```python
from build123d import *

# Parameters (mm, degrees)
F1_DEPTH = 25.4
F2_R     = 6.35
F3_DEPTH = 52.07
F5_DEPTH = 48.768
F7_DEPTH = 25.4
F9_DEPTH = 25.4


with BuildPart() as f1:
    # F0 (on Front) → F1 (new body)
    with BuildSketch(Plane.XZ):
        Polygon((0, 38.1), (0, 0), (76.2, 0), (76.2, 12.7), (25.4, 12.7), (25.4, 38.1), align=None)
    extrude(amount=-F1_DEPTH)

    # F2 (on face) → F3 (cut)
    with BuildSketch(Plane.XZ):
        with Locations((12.7231444902, 26.1663774417)):
            Circle(F2_R)
    extrude(amount=-F3_DEPTH, mode=Mode.SUBTRACT)

    # F4 (on face) → F5 (cut)
    with BuildSketch(Plane.XZ):
        with BuildLine():
            ThreePointArc((12.7, 38.1), (21.6802561211, 34.3802561211), (25.4, 25.4))
            Line((25.4, 25.4), (25.4, 38.1))
            Line((25.4, 38.1), (12.7, 38.1))
        make_face()
        with BuildLine():
            ThreePointArc((0, 25.4), (3.7197438789, 34.3802561211), (12.7, 38.1))
            Line((12.7, 38.1), (0, 38.1))
            Line((0, 38.1), (0, 25.4))
        make_face()
    extrude(amount=-F5_DEPTH, mode=Mode.SUBTRACT)

    # F6 (on face) → F7 (cut)
    with BuildSketch(Plane.XY.offset(12.7)):
        with BuildLine():
            Line((63.5, 19.05), (38.1, 19.05))
            ThreePointArc((38.1, 19.05), (31.75, 12.7), (38.1, 6.35))
            Line((38.1, 6.35), (63.5, 6.35))
            ThreePointArc((63.5, 6.35), (69.85, 12.7), (63.5, 19.05))
        make_face()
    extrude(amount=-F7_DEPTH, mode=Mode.SUBTRACT)

    # F8 (on face) → F9 (cut)
    with BuildSketch(Plane.XY.offset(12.7)):
        with BuildLine():
            ThreePointArc((63.5, 25.4), (72.4802561211, 21.6802561211), (76.2, 12.7))
            Line((76.2, 12.7), (76.2, 25.4))
            Line((76.2, 25.4), (63.5, 25.4))
        make_face()
        with BuildLine():
            ThreePointArc((76.2, 12.7), (72.4802561211, 3.7197438789), (63.5, 0))
            Line((63.5, 0), (76.2, 0))
            Line((76.2, 0), (76.2, 12.7))
        make_face()
    extrude(amount=-F9_DEPTH, mode=Mode.SUBTRACT)


solid = f1.part
```
Here's how the part is built. I have some questions about the finished solid (model axes, mm). A direction names the side the tool comes from. Round coordinates to 2 decimals unless told otherwise and drop trailing zeros. Write each loop counter-clockwise with the first axis right and the second up, starting at its lowest first coordinate (ties: lowest second). Pieces come first, ordered by that corner, then holes. Notation, with made-up numbers: M -5.5,-17 L 46.5,-17 A22 ccw 46.5,-5 Z; hole C -38.5,-16 d8. An arc over 180 degrees is marked long. Answer as CSV lines item,"result". Start each with the question number.
1. Suppose I cut it at A-A on y = 16.75. Write out the boundary of the cut face in (x, z), then the cut area to 3 significant figures.
2. Suppose I cut it at D-D on y = 4.25. Write out the boundary of the cut face in (x, z).
3. I need wall thicknesses on probe 1 along Y at (x, z) = (49, 8.5); probe 2 along Z at (x, y) = (12, 4); probe 3 along X at (y, z) = (20.75, 28). Which ranges of each line are inside material? Lowest first, please.
4. Thinking about a two-plate mould opening in X: for faces 1 (the cylindrical face through (69.85, 12.56, 6.44)), 2 (the flat face through (25.4, 13, 19)), 3 (the flat face through (29, 13, 0)), which applies, released by +X, released by -X, zero draft, split by the parting line, or undercut?
5. On a 3-axis mill with a long thin cutter (end or side, diameter ignored), from which of +Z, -Z, +X, -X, +Y, -Y can I reach the whole of each face in a straight line? I mean faces 4 (the flat face through (51, 4, 12.7)), 5 (the flat face through (51, 19.05, 6)), 6 (the flat face through (24, 0, 15)). Say none if no direction works.
6. Suppose I cut it at C-C on z = 10. Write out the boundary of the cut face in (x, y).
7. Suppose I cut it at B-B on x = 49. Write out the boundary of the cut face in (y, z).
8. I'm going to push flat-ended pins straight in: pin 1 Ø14.5 at (x, z) = (12.72, 26.17) entering from +Y; pin 2 Ø12.5 at (x, y) = (42, 15.5) entering from +Z. Where does each tip first touch, or does it pass through?
Check result:
1,outline,"M 0,0 L 33.21,0 L 33.21,12.7 L 25.4,12.7 L 25.4,25.4 A12.7 ccw 0,25.4 Z; M 68.39,0 L 75.54,0 L 75.54,12.7 L 68.39,12.7 Z; hole C 12.72,26.17 d12.7"
1,area,"962 mm2"
2,outline,"M 0,0 L 72.98,0 L 72.98,12.7 L 25.4,12.7 L 25.4,25.4 A12.7 ccw 0,25.4 Z; hole C 12.72,26.17 d12.7"
3,probe 1,"y = 0 to 6.35, 19.05 to 25.4"
3,probe 2,"z = 0 to 19.86, 32.48 to 38.08"
3,probe 3,"x = 0.27 to 6.64, 18.8 to 25.13"
4,face 1,"undercut"
4,face 2,"released by +X"
4,face 3,"zero draft"
5,face 4,"+Z, +X, +Y, -Y"
5,face 5,"+Z, -Z"
5,face 6,"+Z, -Z, +X, -X, -Y"
6,outline,"M 0,0 L 63.5,0 A12.7 ccw 63.5,25.4 L 0,25.4 Z; hole M 38.1,6.35 L 63.5,6.35 A6.35 ccw 63.5,19.05 L 38.1,19.05 A6.35 ccw Z"
7,outline,"M 0,0 L 6.35,0 L 6.35,12.7 L 0,12.7 Z; M 19.05,0 L 25.4,0 L 25.4,12.7 L 19.05,12.7 Z"
8,pin 1,"stops at y = 25.4"
8,pin 2,"stops at z = 12.7"
